Verification items for the finished model (mm, model axes). Face numbers are marked on the shaded views. A direction names the side the tool comes from. Coordinates: 2 decimals unless noted, no trailing zeros. Write each loop counter-clockwise with the first axis right and the second up, starting at its lowest first coordinate (ties: lowest second). Pieces come first, ordered by that corner, then holes. Notation, with made-up numbers: (73, 88) -> (114, 88) arc R20 ccw to (114, 113) -> close; hole circle Ø3 at (-16, 40). An arc over 180 degrees is marked (long way). Answer in a Markdown table with one row per item.
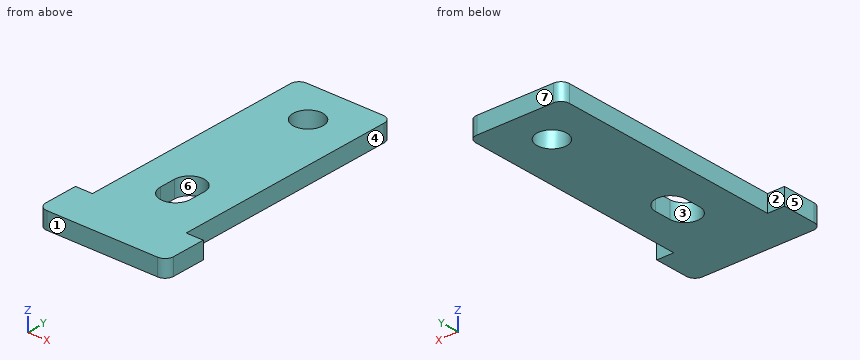
```python
from build123d import *

# Parameters (mm, degrees)
IZIM1_R                     = 1.75
Y_KSEKLIK_EKSTR_ZYON1_DEPTH = 2


with BuildPart() as part:
    # Çizim1 → Yükseklik-Ekstrüzyon1 (new body)
    with BuildSketch(Plane.XY):
        with BuildLine():
            Line((-4.459459459, -15.675675676), (-6.459459459, -15.675675676))
            Line((-6.459459459, -15.675675676), (-6.459459459, -19.675675676))
            ThreePointArc((-6.459459459, -19.675675676), (-6.166566241, -20.382782457), (-5.459459459, -20.675675676))
            Line((-5.459459459, -20.675675676), (7.540540541, -20.675675676))
            ThreePointArc((7.540540541, -20.675675676), (8.247647322, -20.382782457), (8.540540541, -19.675675676))
            Line((8.540540541, -19.675675676), (8.540540541, -15.675675676))
            Line((8.540540541, -15.675675676), (6.540540541, -15.675675676))
            Line((6.540540541, -15.675675676), (6.540540541, 11.024324324))
            ThreePointArc((6.540540541, 11.024324324), (6.247647322, 11.731431106), (5.540540541, 12.024324324))
            Line((5.540540541, 12.024324324), (-3.459459459, 12.024324324))
            ThreePointArc((-3.459459459, 12.024324324), (-4.166566241, 11.731431106), (-4.459459459, 11.024324324))
            Line((-4.459459459, 11.024324324), (-4.459459459, -15.675675676))
        make_face()
        with Locations((1.040540541, 7.074324324)):
            Circle(IZIM1_R, mode=Mode.SUBTRACT)
        with BuildLine():
            Line((-0.709459459, -10.825675676), (-0.709459459, -8.925675676))
            ThreePointArc((-0.709459459, -8.925675676), (1.040540541, -7.175675676), (2.790540541, -8.925675676))
            Line((2.790540541, -8.925675676), (2.790540541, -10.825675676))
            ThreePointArc((2.790540541, -10.825675676), (1.040540541, -12.575675676), (-0.709459459, -10.825675676))
        make_face(mode=Mode.SUBTRACT)
    extrude(amount=Y_KSEKLIK_EKSTR_ZYON1_DEPTH)


solid = part.part
```
1. Mould release check, pull along X, two halves, no side actions. Record for the marked faces 4, 5, 6 and 7: released by +X, released by -X, zero draft, split by the parting line, or undercut.
Geometry says:
| item | result |
|---|---|
| face 4 | released by +X |
| face 5 | released by -X |
| face 6 | undercut |
| face 7 | zero draft |
2. Thickness scan on line 1 (Y direction, x = 2.5, z = 1.6); line 2 (Y direction, x = 2, z = 1.35); line 3 (X direction, y = -9, z = 1.75). Record the ranges inside material, lowest first. Write a range as from..to.
Geometry says:
| item | result |
|---|---|
| line 1 | -20.68..-11.79, -7.96..6.11, 8.04..12.02 |
| line 2 | -20.68..-12.29, -7.46..5.61, 8.54..12.02 |
| line 3 | -4.46..-0.71, 2.79..6.54 |
3. Section check D-D, the plane y = -3.5. Record the boundary of the cut face in (x, z), plus the area to 3 significant figures.
Geometry says:
| item | result |
|---|---|
| outline | (-4.46, 0) -> (6.54, 0) -> (6.54, 2) -> (-4.46, 2) -> close |
| area | 22.0 mm^2 |
4. Depth check by flat-ended pin: P1, Ø1, axis at y = -4, z = 0.5, coming from the -X side. Enter the tip coordinate at first touch or a pass-through.
Geometry says:
| item | result |
|---|---|
| P1 | x = -4.46 |
5. Section check C-C, the plane y = -12. Record the boundary of the cut face in (x, z).
Geometry says:
| item | result |
|---|---|
| outline | (-4.46, 0) -> (-0.26, 0) -> (-0.26, 2) -> (-4.46, 2) -> close; (2.34, 0) -> (6.54, 0) -> (6.54, 2) -> (2.34, 2) -> close |
6. Section check B-B, the plane x = 0. Record the boundary of the cut face in (y, z), plus the area to 3 significant figures.
Geometry says:
| item | result |
|---|---|
| outline | (-20.68, 0) -> (-12.23, 0) -> (-12.23, 2) -> (-20.68, 2) -> close; (-7.52, 0) -> (5.67, 0) -> (5.67, 2) -> (-7.52, 2) -> close; (8.48, 0) -> (12.02, 0) -> (12.02, 2) -> (8.48, 2) -> close |
| area | 50.3 mm^2 |
7. Section check A-A, the plane z = 0.45. Record the boundary of the cut face in (x, y), plus the area to 3 significant figures.
Geometry says:
| item | result |
|---|---|
| outline | (-6.46, -19.68) arc R1 ccw to (-5.46, -20.68) -> (7.54, -20.68) arc R1 ccw to (8.54, -19.68) -> (8.54, -15.68) -> (6.54, -15.68) -> (6.54, 11.02) arc R1 ccw to (5.54, 12.02) -> (-3.46, 12.02) arc R1 ccw to (-4.46, 11.02) -> (-4.46, -15.68) -> (-6.46, -15.68) -> close; hole (-0.71, -10.83) arc R1.75 ccw to (2.79, -10.83) -> (2.79, -8.93) arc R1.75 ccw to (-0.71, -8.93) -> close; hole circle Ø3.5 at (1.04, 7.07) |
| area | 353 mm^2 |
8. Tool access check on the marked faces 1, 2 and 3. Record the directions out of +Z, -Z, +X, -X, +Y, -Y that give a thin tool (end or side, any length) a straight path to the whole face; none if there is none.
Geometry says:
| item | result |
|---|---|
| face 1 | +Z, -Z, +X, -X, -Y |
| face 2 | +Z, -Z, -X, +Y |
| face 3 | +Z, -Z |
